Here's how the part is built. I have some questions about the finished solid (model axes, mm). Face numbers are marked on the shaded views. A direction names the side the tool comes from. Give positions to 0.01 mm unless a question says otherwise; leave off trailing zeros. Write each loop counter-clockwise with the first axis right and the second up, starting at its lowest first coordinate (ties: lowest second). Pieces come first, ordered by that corner, then holes. Notation, with made-up numbers: (-18, -18) - (-8, -18) arc R25 ccw to (-8, -2) - close; hole circle Ø5 at (67, -15.5). An arc over 180 degrees is marked (long way). Use a Markdown table: item, result.
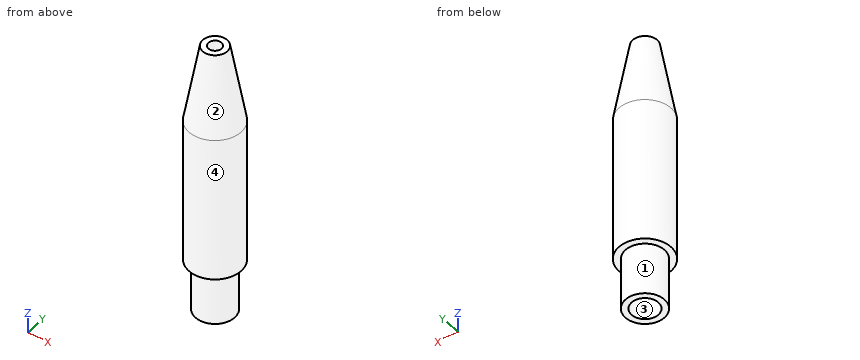
```python
from build123d import *

# Parameters (mm, degrees)
SKETCH1_R                       = 6.35
BOSS_EXTRUDE1_DEPTH             = 67.31
SKETCH8_R                       = 1.5875
CUT_EXTRUDE1_DEPTH              = 68.31
SKETCH10_R                      = 6.35
SKETCH10_R_2                    = 4.7625
CUT_EXTRUDE2_DEPTH              = 12.7
F_1_4_0_25_DIAMETER_HOLE1_D     = 6.5278
F_1_4_0_25_DIAMETER_HOLE1_DEPTH = 59.69
F_1_4_0_25_DIAMETER_HOLE1_TIP   = 1.961148974


with BuildPart() as part:
    # Sketch1 → Boss-Extrude1 (new body)
    with BuildSketch(Plane.XY):
        Circle(SKETCH1_R)
    extrude(amount=BOSS_EXTRUDE1_DEPTH)

    # Sketch7 → Cut-Revolve1 (revolve, cut)
    with BuildSketch(Plane(origin=(0, 0, 0), x_dir=(1, 0, 0), z_dir=(0, 1, 0))):
        Polygon((6.35, -67.31), (6.35, -48.26), (2.990971018, -67.31), align=None)
    revolve(axis=Axis((0, 0, -47.573976859), (0, 0, 1)), mode=Mode.SUBTRACT)

    # Sketch8 → Cut-Extrude1 (cut, through all)
    with BuildSketch(Plane.XY.offset(67.31)):
        Circle(SKETCH8_R)
    extrude(amount=-CUT_EXTRUDE1_DEPTH, mode=Mode.SUBTRACT)

    # Sketch10 → Cut-Extrude2 (cut)
    with BuildSketch(Plane(origin=(0, 0, 0), x_dir=(-1, 0, 0), z_dir=(0, 0, -1))):
        Circle(SKETCH10_R)
        Circle(SKETCH10_R_2, mode=Mode.SUBTRACT)
    extrude(amount=-CUT_EXTRUDE2_DEPTH, mode=Mode.SUBTRACT)

    # 1/4 (0.25) Diameter Hole1
    with Locations(Plane(origin=(0, 0, 0), x_dir=(-1, 0, 0), z_dir=(0, 0, -1))):
        with Locations((0, 0)):
            Hole(F_1_4_0_25_DIAMETER_HOLE1_D / 2, depth=F_1_4_0_25_DIAMETER_HOLE1_DEPTH)
            with Locations((0, 0, -(F_1_4_0_25_DIAMETER_HOLE1_DEPTH + F_1_4_0_25_DIAMETER_HOLE1_TIP / 2))):  # 118° drill point
                Cone(0, F_1_4_0_25_DIAMETER_HOLE1_D / 2, F_1_4_0_25_DIAMETER_HOLE1_TIP, mode=Mode.SUBTRACT)


solid = part.part
```
Item 1: Will this pin go through, and if not, where does the flat tip stop? pin 1 Ø5 at (x, y) = (0, 0) entering from -Z.
Values:
| item | result |
|---|---|
| pin 1 | stops at z = 60.15 |
Item 2: I need wall thicknesses on line 1 along Y through (x, z) = (0, 30); line 2 along X through (y, z) = (0, 65.75); line 3 along Y through (x, z) = (0, 12). Which ranges of each line are inside material? Lowest first, please. Write a range as [from, to].
Values:
| item | result |
|---|---|
| line 1 | y = [-6.35, -3.26], [3.26, 6.35] |
| line 2 | x = [-3.27, -1.59], [1.59, 3.27] |
| line 3 | y = [-4.76, -3.26], [3.26, 4.76] |
Item 3: Thinking about a two-plate mould opening in X: for the marked faces 3 and 4, which applies, +X half, -X half, draft (parallel to the pull), parting line (faces both ways), or undercut?
Values:
| item | result |
|---|---|
| face 3 | undercut |
| face 4 | parting line |
Item 4: For the marked faces 1 and 2, which set-ups out of +Z, -Z, +X, -X, +Y, -Y let a thin tool reach every point of the face, with its end or its side?
Values:
| item | result |
|---|---|
| face 1 | -Z |
| face 2 | +Z |
Item 5: If we section it at A-A, the plane x = 0: Write out the boundary of the cut face in (y, z).
Values:
| item | result |
|---|---|
| outline | (-6.35, 12.7) - (-4.76, 12.7) - (-4.76, 0) - (-3.26, 0) - (-3.26, 59.69) - (-1.59, 60.7) - (-1.59, 67.31) - (-2.99, 67.31) - (-6.35, 48.26) - close; (1.59, 60.7) - (3.26, 59.69) - (3.26, 0) - (4.76, 0) - (4.76, 12.7) - (6.35, 12.7) - (6.35, 48.26) - (2.99, 67.31) - (1.59, 67.31) - close |
Item 6: If we section it at C-C, the plane z = 24: Write out the boundary of the cut face in (x, y), plus the area to 3 significant figures.
Values:
| item | result |
|---|---|
| outline | circle Ø12.7 at (0, 0); hole circle Ø6.53 at (0, 0) |
| area | 93.2 mm2 |
